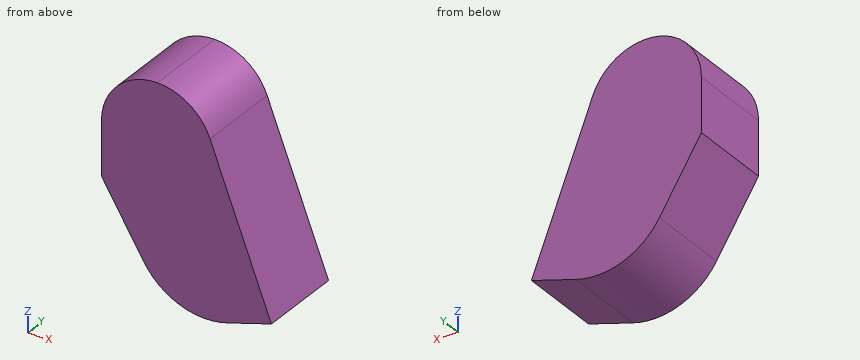
from build123d import *

# Parameters (mm, degrees)
BOSS_EXTRUDE1_DEPTH = 58.42
FILLET3_R           = 39.603164


with BuildPart() as part:
    # Sketch1 → Boss-Extrude1 (new body)
    with BuildSketch(Plane(origin=(0, 0, 0), x_dir=(1, 0, 0), z_dir=(0, 1, 0))):
        with BuildLine():
            Line((-66.673768512, 0), (-37.067821873, 47.633329988))
            ThreePointArc((-37.067821873, 47.633329988), (-11.329209284, 68.541566023), (21.82652777, 69.113940477))
            Line((21.82652777, 69.113940477), (53.138492197, 58.903517294))
            Line((53.138492197, 58.903517294), (0, -77.45185891))
            Line((0, -77.45185891), (-66.673768512, -77.45185891))
            Line((-66.673768512, -77.45185891), (-66.673768512, 0))
        make_face()
    extrude(amount=BOSS_EXTRUDE1_DEPTH)

    # Fillet3
    fillet3_edges = [part.edges().sort_by_distance(p)[0] for p in [
        (0, 29.21, 77.45185891),
        (-66.673768512, 29.21, 77.45185891),
    ]]
    fillet(fillet3_edges, radius=FILLET3_R)


solid = part.part
Geometry: final body of the model. Coordinates: model frame, mm. Coordinates: 2 decimals unless noted, no trailing zeros. Order: outer loops, then holes, each group sorted by start corner. A loop starts at its lowest first (then second) coordinate and runs counter-clockwise, first axis right, second up.
(1) Section query A-A (y = 12.5). Return the cut outline in (x, z).
(2) Section query B-B (z = -33.5). Return the cut outline in (x, y), plus the area to 3 significant figures.
(3) Section query C-C (x = -10). Return the cut outline in (y, z), plus the area to 3 significant figures.
(4) Material intervals for probe 1 along Z at (x, y) = (-27.5, 35); probe 2 along X at (y, z) = (29, -34); probe 3 along X at (y, z) = (9.5, 55.5), sorted ascending.
(5) First-contact query: pin 1 (1 mm diameter, centred on x = 13.5, z = 29, fed in from -Y); pin 2 (8 mm diameter, centred on y = 32.5, z = 42.5, fed in from -X); pin 3 (1 mm diameter, centred on y = 38.5, z = -11, fed in from +X); pin 4 (3 mm diameter, centred on y = 50.5, z = -21.5, fed in from +X). Flat tips, straight axial feed; report the tip coordinate or a pass-through.
Solution:
1. outline: (-66.67, 0) - (-37.07, -47.63) arc R50.8 ccw to (21.83, -69.11) - (53.14, -58.9) - (9.83, 52.23) arc R39.6 ccw to (-66.67, 37.85) - close
2. outline: (-45.85, 0) - (43.24, 0) - (43.24, 58.42) - (-45.85, 58.42) - close
2. area: 5,200 mm2
3. outline: (0, -69.01) - (58.42, -69.01) - (58.42, 73.58) - (0, 73.58) - close
3. area: 8,330 mm2
4. probe 1: z = -58.94 to 77.45
4. probe 2: x = -45.54 to 43.43
4. probe 3: x = -62.52 to 8.38
5. pin 1: stops at y = 0
5. pin 2: stops at x = -66.67
5. pin 3: stops at x = 34.67
5. pin 4: stops at x = 39.15
